The figure shows three views and two pictorial views of one solid part (mm, origin at its lowest corner). Answer the questions. A direction names the side the tool comes from. Round coordinates to 2 decimals unless told otherwise and drop trailing zeros. Order: outer loops, then holes, each group sorted by start corner. A loop starts at its lowest first (then second) coordinate and runs counter-clockwise, first axis right, second up.
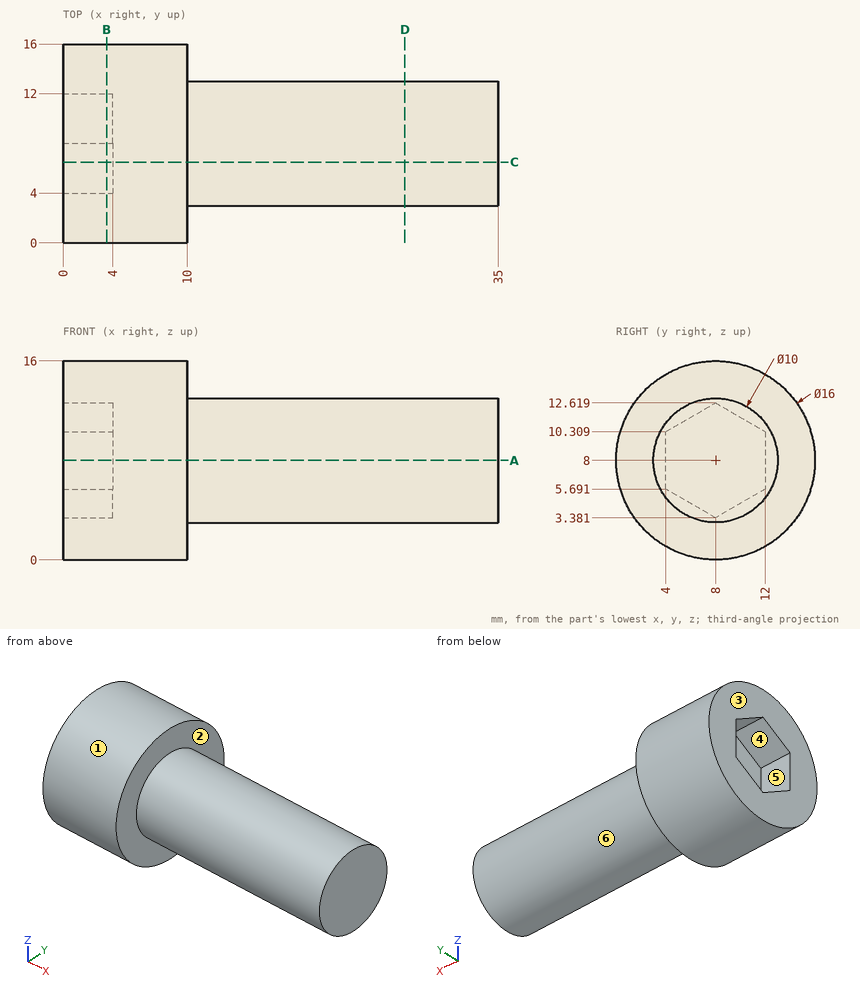
Item 1: Given pin 1 (5 mm diameter, centred on x = 5.5, z = 2, fed in from +Y); pin 2 (5 mm diameter, centred on x = 31, y = 2.5, fed in from -Z); pin 3 (1.5 mm diameter, centred on x = 12.5, z = 7.5, fed in from +Y), each flat-ended and moving along its own axis, determine where each tip first touches the part or whether it passes through.
Item 2: Find section A-A (z = 8). Write down the section's boundary in (x, y), plus the area to 3 significant figures.
Item 3: Find section C-C (y = 6.5). Write down the section's boundary in (x, z), plus the area to 3 significant figures.
Item 4: Find section B-B (x = 3.5). Write down the section's boundary in (y, z), plus the area to 3 significant figures.
Item 5: For a pull along Y with two mould halves and no side action, classify the marked faces 3, 4, 5 and 6 as released by +Y, released by -Y, zero draft, split by the parting line, or undercut.
Item 6: Find section D-D (x = 27.5). Write down the section's boundary in (y, z).
Item 7: Find the intervals of material crossed by line 1 along X through (y, z) = (10.5, 3.5); line 2 along X through (y, z) = (8.75, 7); line 3 along Y through (x, z) = (20.5, 8), in increasing order.
Item 8: A tool of negligible diameter and unlimited length cuts with its end or side. For the marked faces 1 and 2, from which of +Z, -Z, +X, -X, +Y, -Y can it reach the whole face along a straight path? Write none if from no direction.
Model answer:
1. pin 1: stops at y = 15.19
1. pin 2: stops at z = 4
1. pin 3: stops at y = 13
2. outline: (0, 0) - (10, 0) - (10, 3) - (35, 3) - (35, 13) - (10, 13) - (10, 16) - (0, 16) - (0, 12) - (4, 12) - (4, 4) - (0, 4) - close
2. area: 378 mm2
3. outline: (0, 0.14) - (10, 0.14) - (10, 3.23) - (35, 3.23) - (35, 12.77) - (10, 12.77) - (10, 15.86) - (0, 15.86) - (0, 11.75) - (4, 11.75) - (4, 4.25) - (0, 4.25) - close
3. area: 366 mm2
4. outline: circle Ø16 at (8, 8); hole (4, 5.69) - (8, 3.38) - (12, 5.69) - (12, 10.31) - (8, 12.62) - (4, 10.31) - close
4. area: 146 mm2
5. face 3: zero draft
5. face 4: undercut
5. face 5: undercut
5. face 6: split by the parting line
6. outline: circle Ø10 at (8, 8)
7. line 1: x = 0 to 10
7. line 2: x = 4 to 35
7. line 3: y = 3 to 13
8. face 1: +X, -X
8. face 2: +X
